The model under review builds one solid part; all positions refer to its coordinate system, in mm. A direction names the side the tool comes from. Coordinates: 2 decimals unless noted, no trailing zeros. Order: outer loops, then holes, each group sorted by start corner. A loop starts at its lowest first (then second) coordinate and runs counter-clockwise, first axis right, second up. Notation, with made-up numbers: (-12, -30.75) -> (5, -30.75) arc R33 ccw to (5, 2.25) -> close; hole circle Ø1 at (-10.5, -28). An arc over 180 degrees is marked (long way). Use CSV: the item, a comma, the result in double quotes. Start each with the question number.
```python
from build123d import *

# Parameters (mm, degrees)
BOSS_EXTRU_1_DEPTH      = 22
ENL_V_MAT_EXTRU_1_REACH = 35.355
ESQUISSE2_W             = 5
ESQUISSE2_H             = 31.584947586
ESQUISSE3_R             = 1.25
ENL_V_MAT_EXTRU_2_DEPTH = 4
ENL_V_MAT_EXTRU_3_REACH = 68
ESQUISSE5_R             = 2.5


with BuildPart() as part:
    # Esquisse1 → Boss.-Extru.1 (new body)
    with BuildSketch(Plane.XY):
        with BuildLine():
            Line((0, 0), (0, 5))
            ThreePointArc((0, 5), (16.362517736, 18.234357648), (26.664753317, 36.584947586))
            ThreePointArc((26.664753317, 36.584947586), (26.318927206, 39.062275696), (24, 40))
            Line((24, 40), (24, 70))
            Line((24, 70), (27, 70))
            Line((27, 70), (33.355191258, 43.816329185))
            ThreePointArc((33.355191258, 43.816329185), (27.670942171, 21.661025112), (12, 5))
            Line((12, 5), (12, 0))
            Line((12, 0), (0, 0))
        make_face()
    extrude(amount=BOSS_EXTRU_1_DEPTH)

    # Esquisse2 → Enlèv. mat.-Extru.1 (cut, up to next)
    with BuildSketch(Plane.ZY, mode=Mode.PRIVATE) as enl_v_mat_extru_1_sk1:
        with Locations((2.5, 20.792473793)):
            Rectangle(ESQUISSE2_W, ESQUISSE2_H)
    enl_v_mat_extru_1_tool1 = extrude(enl_v_mat_extru_1_sk1.sketch, amount=-ENL_V_MAT_EXTRU_1_REACH, mode=Mode.PRIVATE) & part.part
    add(enl_v_mat_extru_1_tool1.solids().sort_by_distance((0, 20.792474, 2.5))[0], mode=Mode.SUBTRACT)
    # Esquisse2 → Enlèv. mat.-Extru.1 (cut, up to next)
    with BuildSketch(Plane.ZY, mode=Mode.PRIVATE) as enl_v_mat_extru_1_sk2:
        with Locations((19.5, 20.792473793)):
            Rectangle(ESQUISSE2_W, ESQUISSE2_H)
    enl_v_mat_extru_1_tool2 = extrude(enl_v_mat_extru_1_sk2.sketch, amount=-ENL_V_MAT_EXTRU_1_REACH, mode=Mode.PRIVATE) & part.part
    add(enl_v_mat_extru_1_tool2.solids().sort_by_distance((0, 20.792474, 19.5))[0], mode=Mode.SUBTRACT)

    # Esquisse3 → Enlèv. mat.-Extru.2 (cut)
    with BuildSketch(Plane.XZ):
        with Locations((6, 18.5)):
            Circle(ESQUISSE3_R)
        with Locations((6, 3.5)):
            Circle(ESQUISSE3_R)
    extrude(amount=-ENL_V_MAT_EXTRU_2_DEPTH, mode=Mode.SUBTRACT)

    # Esquisse5 → Enlèv. mat.-Extru.3 (cut, up to next)
    with BuildSketch(Plane(origin=(0, 4, 0), x_dir=(-1, 0, 0), z_dir=(0, -1, 0)), mode=Mode.PRIVATE) as enl_v_mat_extru_3_sk1:
        with Locations((-6, -3.5)):
            Circle(ESQUISSE5_R)
    enl_v_mat_extru_3_tool1 = extrude(enl_v_mat_extru_3_sk1.sketch, amount=-ENL_V_MAT_EXTRU_3_REACH, mode=Mode.PRIVATE) & part.part
    add(enl_v_mat_extru_3_tool1.solids().sort_by_distance((6, 4, 3.5))[0], mode=Mode.SUBTRACT)
    # Esquisse5 → Enlèv. mat.-Extru.3 (cut, up to next)
    with BuildSketch(Plane(origin=(0, 4, 0), x_dir=(-1, 0, 0), z_dir=(0, -1, 0)), mode=Mode.PRIVATE) as enl_v_mat_extru_3_sk2:
        with Locations((-6, -18.5)):
            Circle(ESQUISSE5_R)
    enl_v_mat_extru_3_tool2 = extrude(enl_v_mat_extru_3_sk2.sketch, amount=-ENL_V_MAT_EXTRU_3_REACH, mode=Mode.PRIVATE) & part.part
    add(enl_v_mat_extru_3_tool2.solids().sort_by_distance((6, 4, 18.5))[0], mode=Mode.SUBTRACT)


solid = part.part
```
Q1. For faces 4 (the flat face through (5.9, 5, 0.8)), 5 (the flat face through (30, 36.585, 19)), 6 (the flat face through (24, 55, 11)), list the 3-axis set-ups (+Z, -Z, +X, -X, +Y, -Y) from which the entire face can be reached by the end or side of a thin tool; tool diameter is ignored.
Q2. Add section A-A, the plane z = 18.5. State the section outline as (x, y) points, then the cut area to 3 significant figures.
Q3. Add section C-C, the plane x = 6. State the section outline as (y, z) points.
Q4. Clearance check with flat-ended pins moving along their axes: pin 1 Ø2 at (x, z) = (6, 3.5) entering from -Y; pin 2 Ø1 at (x, y) = (15, 16) entering from -Z; pin 3 Ø12 at (x, z) = (19, 14) entering from -Y; pin 4 Ø4 at (x, z) = (7.5, 20) entering from +Y. State where each tip first meets the part, or that it passes through.
Q5. Add section B-B, the plane z = 10. State the section outline as (x, y) points.
Q6. Add section D-D, the plane y = 9. State the section outline as (x, z) points.
Q7. To check wall thickness, follow probe 1 along Z at (x, y) = (6, 2); probe 2 along Y at (x, z) = (8.5, 19); probe 3 along Z at (x, y) = (6, 5.5). State the ranges of each line that lie inside material, in increasing order.
Q8. Draft analysis for pull direction Y (two halves, no side actions). For faces 1 (the cylindrical face through (26.341, 39.033, 10.846)), 2 (the flat face through (5, 4, 17)), 3 (the flat face through (6, 3, 22)), state which applies: +Y half, -Y half, draft (parallel to the pull), parting line (faces both ways), or undercut.
Answer block:
1,face 4,"-Z, +X, -X, +Y"
1,face 5,"+Z, +X, -X, -Y"
1,face 6,"+Z, -Z, -X, +Y"
2,outline,"(0, 0) -> (4.75, 0) -> (4.75, 4) -> (3.5, 4) -> (3.5, 5) -> (0, 5) -> close; (7.25, 0) -> (12, 0) -> (12, 5) -> (8.5, 5) -> (8.5, 4) -> (7.25, 4) -> close; (24, 40) arc R2.5 cw to (26.66, 36.58) -> (32.79, 36.58) arc R45.9 ccw to (33.36, 43.82) -> (27, 70) -> (24, 70) -> close"
2,area,"265 mm²"
3,outline,"(0, 0) -> (5, 0) -> (5, 1) -> (4, 1) -> (4, 2.25) -> (0, 2.25) -> close; (0, 4.75) -> (4, 4.75) -> (4, 6) -> (8.71, 6) -> (8.71, 16) -> (4, 16) -> (4, 17.25) -> (0, 17.25) -> close; (0, 19.75) -> (4, 19.75) -> (4, 21) -> (5, 21) -> (5, 22) -> (0, 22) -> close"
4,pin 1,"passes through"
4,pin 2,"stops at z = 5"
4,pin 3,"stops at y = 5.65"
4,pin 4,"stops at y = 5"
5,outline,"(0, 0) -> (12, 0) -> (12, 5) arc R45.9 ccw to (33.36, 43.82) -> (27, 70) -> (24, 70) -> (24, 40) arc R2.5 cw to (26.66, 36.58) arc R55.84 cw to (0, 5) -> close"
6,outline,"(6.41, 5.97) arc R2.5 cw to (8, 5) -> (17.4, 5) -> (17.4, 17) -> (8, 17) arc R2.5 cw to (6.41, 16.03) -> close"
7,probe 1,"z = 0 to 2.25, 4.75 to 17.25, 19.75 to 22"
7,probe 2,"y = 0 to 5"
7,probe 3,"z = 6 to 16"
8,face 1,"undercut"
8,face 2,"+Y half"
8,face 3,"draft"
